Part model, mm, in its own coordinate system. Give positions to 0.01 mm unless a question says otherwise; leave off trailing zeros. Write each loop counter-clockwise with the first axis right and the second up, starting at its lowest first coordinate (ties: lowest second). Pieces come first, ordered by that corner, then holes. Notation, with made-up numbers: M -31,85 L 9,85 A19 ccw 9,99 Z; hole C 7.25,28.25 d5. An arc over 180 degrees is marked long. Use a Markdown table: item, result. Add a question column.
from build123d import *

# Parameters (mm, degrees)
SKETCH3_W            = 152.4
SKETCH3_H            = 19.05
BASE_FLANGE1_DEPTH   = 1.5748
EDGE_FLANGE1_DEPTH   = 101.6
M6_CLEARANCE_HOLE1_D = 6.6


# Sheet-metal steps are written as plain solids
with BuildPart() as part:
    # Sketch3 → Base-Flange1 (new body)
    with BuildSketch(Plane.XY):
        Rectangle(SKETCH3_W, SKETCH3_H)
    extrude(amount=-BASE_FLANGE1_DEPTH)

    # Edge-Flange1 section (across the edge) → Edge-Flange1 (add)
    with BuildSketch(Plane(origin=(50.8, 11.30330971, 0), x_dir=(0, -0.7071067811865488, -0.7071067811865464), z_dir=(-1, 0, 0))):
        with BuildLine():
            Line((-1.5748, 1.77830971), (-1.5748, 34.298096482))
            Line((-1.5748, 34.298096482), (0, 34.298096482))
            Line((0, 34.298096482), (0, 1.77830971))
            ThreePointArc((0, 1.77830971), (0.454715384, 1.097780046), (1.257454855, 1.257454855))
            Line((1.257454855, 1.257454855), (2.371006614, 0.143903096))
            ThreePointArc((2.371006614, 0.143903096), (-0.147934486, -0.357145441), (-1.5748, 1.77830971))
        make_face()
    extrude(amount=EDGE_FLANGE1_DEPTH)

    # M6 Clearance Hole1 (through all)
    with Locations(Plane.XY):
        with Locations((-63.5, 0), (63.5, 0)):
            Hole(M6_CLEARANCE_HOLE1_D / 2)


solid = part.part
1. Cut at C-C (y = 8.25). Write the cut outline in (x, z).
2. Cut at A-A (y = 1.75). Write the cut outline in (x, z).
3. Cut at D-D (x = 25). Write the cut outline in (y, z) (3 decimals), then the cut area to 3 significant figures.
4. Drill centre lines: probe 1 along Y at (x, z) = (63.5, -1.2) (3 decimals); probe 2 along X at (y, z) = (3.5, 9); probe 3 along Z at (x, y) = (-31, 5.75). Where is each one in solid material? Low to high. Write a range as [from, to].
5. Mould opens along Z. For faces 1 (the flat face through (-1, 0, 0)), 2 (the cylindrical face through (0.711, 11.646, -0.183)), 3 (the flat face through (0.711, -1.613, 12.916)), 4 (the flat face through (-1, 0, -1.575)) say: released by +Z, released by -Z, zero draft, split by the parting line, or undercut.
6. Flat gauge pins, fed straight in: pin 1 (4 mm diameter, centred on x = -27.5, z = 14, fed in from -Y); pin 2 (10 mm diameter, centred on y = -6.5, z = 22, fed in from -X); pin 3 (4 mm diameter, centred on x = -10.5, y = -9.5, fed in from +Z); pin 4 (4 mm diameter, centred on x = 63.5, y = 0, fed in from -Z). Where does each tip first touch, or does it go through?
7. Cut at B-B (x = -63.5). Write the cut outline in (y, z) (3 decimals), then the cut area to 3 significant figures.
A:
| question | item | result |
|---|---|---|
| 1 | outline | M -76.2,-1.57 L 76.2,-1.57 L 76.2,0 L -76.2,0 Z; M -50.8,3.05 L 50.8,3.05 L 50.8,5.28 L -50.8,5.28 Z |
| 2 | outline | M -76.2,-1.57 L -66.3,-1.57 L -66.3,0 L -76.2,0 Z; M -60.7,-1.57 L 60.7,-1.57 L 60.7,0 L -60.7,0 Z; M -50.8,9.55 L 50.8,9.55 L 50.8,11.78 L -50.8,11.78 Z; M 66.3,-1.57 L 76.2,-1.57 L 76.2,0 L 66.3,0 Z |
| 3 | outline | M -12.949,24.252 L 10.046,1.257 A0.737 cw 9.525,0 L -9.525,0 L -9.525,-1.575 L 9.525,-1.575 A2.311 ccw 11.159,2.371 L -11.836,25.366 Z |
| 3 | area | 86.9 mm² |
| 4 | probe 1 | y = [-9.525, -3.3], [3.3, 9.525] |
| 4 | probe 2 | x = [-50.8, 50.8] |
| 4 | probe 3 | z = [-1.57, 0], [5.55, 7.78] |
| 5 | face 1 | undercut |
| 5 | face 2 | split by the parting line |
| 5 | face 3 | undercut |
| 5 | face 4 | released by -Z |
| 6 | pin 1 | stops at y = -4.7 |
| 6 | pin 2 | stops at x = -50.8 |
| 6 | pin 3 | stops at z = 25.03 |
| 6 | pin 4 | passes through |
| 7 | outline | M -9.525,-1.575 L -3.3,-1.575 L -3.3,0 L -9.525,0 Z; M 3.3,-1.575 L 9.525,-1.575 L 9.525,0 L 3.3,0 Z |
| 7 | area | 19.6 mm² |
